```python
from build123d import *

# Parameters (mm, degrees)
F0_R     = 44.45
F1_DEPTH = 25.4
F2_R     = 40.64
F3_DEPTH = 19.05
F4_R     = 4.445
F5_DEPTH = 25.4


with BuildPart() as f1:
    # F0 (on Front) → F1 (new body)
    with BuildSketch(Plane.XZ):
        Circle(F0_R)
    extrude(amount=F1_DEPTH)

    # F2 (on Front) → F3 (cut)
    with BuildSketch(Plane.XZ):
        Circle(F2_R)
    extrude(amount=F3_DEPTH, mode=Mode.SUBTRACT)

    # F4 (on Front) → F5 (cut)
    with BuildSketch(Plane.XZ):
        with Locations((0, 30.48)):
            Circle(F4_R)
        with Locations((-15.24, 15.24)):
            Circle(F4_R)
        with Locations((-30.48, 0)):
            Circle(F4_R)
        with Locations((15.24, 15.24)):
            Circle(F4_R)
        with Locations((30.48, 0)):
            Circle(F4_R)
        with Locations((-15.24, -15.24)):
            Circle(F4_R)
        with Locations((15.24, -15.24)):
            Circle(F4_R)
        with Locations((0, -30.48)):
            Circle(F4_R)
        Circle(F4_R)
    extrude(amount=F5_DEPTH, mode=Mode.SUBTRACT)


solid = f1.part
```
Can you work these out from the model? Positions are in its coordinate system, mm. A direction names the side the tool comes from. Coordinates: 2 decimals unless noted, no trailing zeros. Loops run counter-clockwise (first coordinate to the right, second up) from the corner with the lowest first, then second, coordinate; pieces in that order, holes last. Notation, with made-up numbers: M -13.75,58 L 11.25,58 A26 cw 11.25,85 Z; hole C 68,49 d1. An arc over 180 degrees is marked long. Put each result on its own line as item: value. Start each with the question number.
(1) Which directions (+Z, -Z, +X, -X, +Y, -Y) give clear straight access to the entire face, cutting with the end or side of a thin tool? Please do faces 1 (the face through (-18.52, -22.18, -12.24)), 2 (the face through (-1, -19.05, -8)).
(2) Imagine slicing it at A-A on z = 0. List the corners of the cut face in (x, y) for me (3 decimals).
(3) I need wall thicknesses on probe 1 along Z at (x, y) = (0, -21.75) (3 decimals); probe 2 along Z at (x, y) = (15.5, -20.5); probe 3 along Z at (x, y) = (15.24, -21.25) (3 decimals). Which ranges of each line are inside material? Lowest first, please.
(4) Imagine slicing it at B-B on x = 30.48. List the corners of the cut face in (y, z) for me (3 decimals).
(5) Imagine slicing it at D-D on z = -15.24. List the corners of the cut face in (x, y) for me (3 decimals).
(6) Imagine slicing it at C-C on x = 15. List the corners of the cut face in (y, z) for me.
(7) Will these pins go through, and if not, where does the flat tip stop? pin 1 Ø4 at (x, y) = (3.5, -11) entering from -Z; pin 2 Ø1 at (y, z) = (-20.5, -17.5) entering from +X; pin 3 Ø11.5 at (x, z) = (15.24, 15.24) entering from +Y; pin 4 Ø8 at (x, z) = (15.24, -15.24) entering from -Y.
(8) We'd pull the mould along X, two halves only. Please class faces 3 (the face through (42.397, -12.522, 13.352)), 4 (the face through (34.586, -22.181, -1.702)), 5 (the face through (-1, -25.4, -9)): +X half, -X half, draft (parallel to the pull), parting line (faces both ways), or undercut.
Worked answers:
1. face 1: +Y, -Y
1. face 2: +Y
2. outline: M -44.45,-25.4 L -34.925,-25.4 L -34.925,-19.05 L -40.64,-19.05 L -40.64,0 L -44.45,0 Z; M -26.035,-25.4 L -4.445,-25.4 L -4.445,-19.05 L -26.035,-19.05 Z; M 4.445,-25.4 L 26.035,-25.4 L 26.035,-19.05 L 4.445,-19.05 Z; M 34.925,-25.4 L 44.45,-25.4 L 44.45,0 L 40.64,0 L 40.64,-19.05 L 34.925,-19.05 Z
3. probe 1: z = -44.45 to -34.925, -26.035 to -4.445, 4.445 to 26.035, 34.925 to 44.45
3. probe 2: z = -41.66 to -19.68, -10.8 to 10.8, 19.68 to 41.66
3. probe 3: z = -41.756 to -19.685, -10.795 to 10.795, 19.685 to 41.756
4. outline: M -25.4,-32.354 L 0,-32.354 L 0,-26.881 L -19.05,-26.881 L -19.05,-4.445 L -25.4,-4.445 Z; M -25.4,4.445 L -19.05,4.445 L -19.05,26.881 L 0,26.881 L 0,32.354 L -25.4,32.354 Z
5. outline: M -41.756,-25.4 L -19.685,-25.4 L -19.685,-19.05 L -37.674,-19.05 L -37.674,0 L -41.756,0 Z; M -10.795,-25.4 L 10.795,-25.4 L 10.795,-19.05 L -10.795,-19.05 Z; M 19.685,-25.4 L 41.756,-25.4 L 41.756,0 L 37.674,0 L 37.674,-19.05 L 19.685,-19.05 Z
6. outline: M -25.4,-41.84 L 0,-41.84 L 0,-37.77 L -19.05,-37.77 L -19.05,-19.68 L -25.4,-19.68 Z; M -25.4,-10.8 L -19.05,-10.8 L -19.05,10.8 L -25.4,10.8 Z; M -25.4,19.68 L -19.05,19.68 L -19.05,37.77 L 0,37.77 L 0,41.84 L -25.4,41.84 Z
7. pin 1: stops at z = -44.42
7. pin 2: stops at x = 41.07
7. pin 3: stops at y = -19.05
7. pin 4: passes through
8. face 3: parting line
8. face 4: undercut
8. face 5: draft
